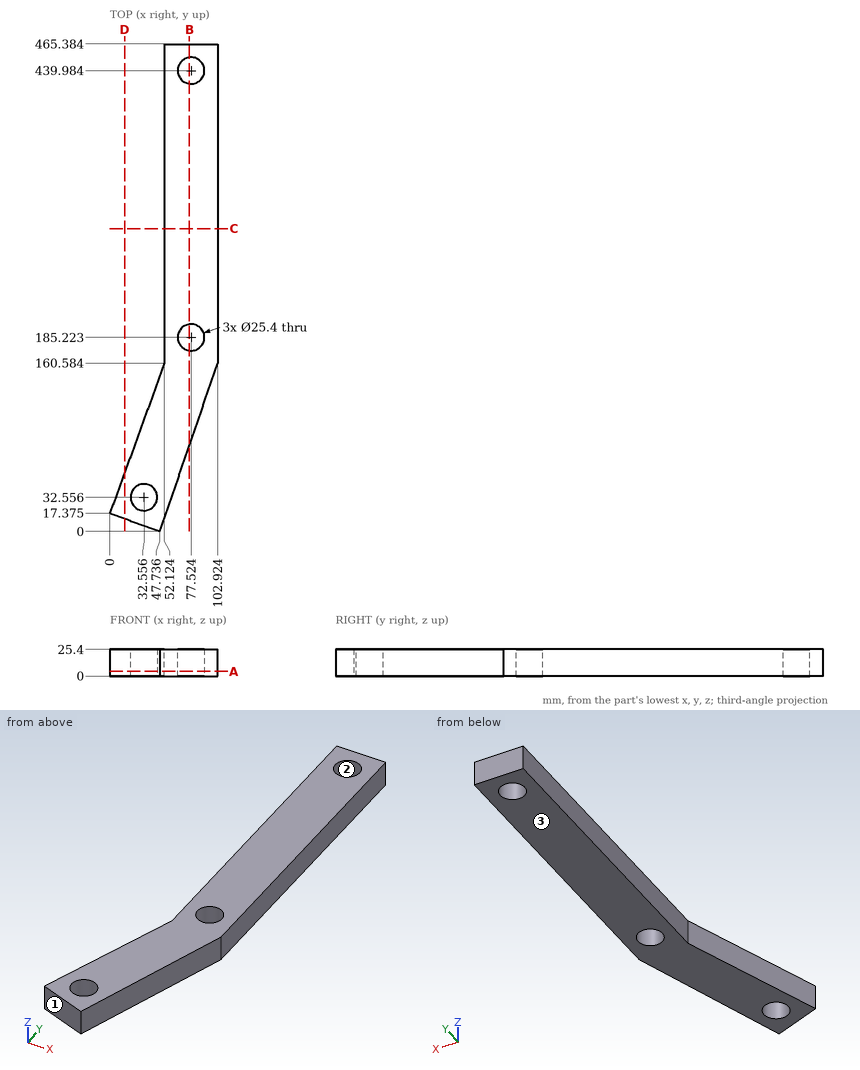
Drawing for the job (mm, zero at the part's lowest x, y, z). Coordinates: 2 decimals unless noted, no trailing zeros. Order: outer loops, then holes, each group sorted by start corner. A loop starts at its lowest first (then second) coordinate and runs counter-clockwise, first axis right, second up. Notation, with made-up numbers: (29.5, 13.5) -> (37.5, 13.5) arc R33 cw to (37.5, 47.5) -> close; hole circle Ø3 at (13.25, 72.5). An arc over 180 degrees is marked (long way). Return JSON: item names as keys, results as strings.
Item 1: Mould opens along X. For the marked faces 1, 2 and 3 say: pulls with the +X half, pulls with the -X half, needs draft (parallel to the pull), parting line crosses it, or undercut.
Model answer:
{"face 1": "pulls with the -X half", "face 2": "undercut", "face 3": "needs draft"}
Item 2: Slice it at D-D (x = 14). Write the cut outline in (y, z), then the cut area to 3 significant figures.
Model answer:
{"outline": "(12.28, 0) -> (55.84, 0) -> (55.84, 25.4) -> (12.28, 25.4) -> close", "area": "1,110 mm²"}
Item 3: Slice it at B-B (x = 76). Write the cut outline in (y, z) (1 decimal).
Model answer:
{"outline": "(82.2, 0) -> (172.6, 0) -> (172.6, 25.4) -> (82.2, 25.4) -> close; (197.8, 0) -> (427.4, 0) -> (427.4, 25.4) -> (197.8, 25.4) -> close; (452.6, 0) -> (465.4, 0) -> (465.4, 25.4) -> (452.6, 25.4) -> close"}
Item 4: Pin check, flat tips, straight feed: P1, Ø2, axis at y = 353.5, z = 15.5, coming from the -X side; P2, Ø3, axis at y = 141.5, z = 14, coming from the +X side. Stop position of each tip, or through.
Model answer:
{"P1": "stops at x = 52.12", "P2": "stops at x = 96.88"}
Item 5: Slice it at C-C (y = 289). Write the cut outline in (x, z).
Model answer:
{"outline": "(52.12, 0) -> (102.92, 0) -> (102.92, 25.4) -> (52.12, 25.4) -> close"}
Item 6: Wall check: line 1 along X through (y, z) = (325.5, 17.5); line 2 along X through (y, z) = (189.5, 23.75) (1 decimal); line 3 along X through (y, z) = (158.5, 7) (1 decimal). Give the ranges that are in metal, low to high. Write a range as from..to.
Model answer:
{"line 1": "x = 52.12..102.92", "line 2": "x = 52.1..65.6, 89.5..102.9", "line 3": "x = 51.4..102.2"}
Item 7: Slice it at A-A (z = 4.5). Write the cut outline in (x, y) (1 decimal).
Model answer:
{"outline": "(0, 17.4) -> (47.7, 0) -> (102.9, 160.6) -> (102.9, 465.4) -> (52.1, 465.4) -> (52.1, 160.6) -> close; hole circle Ø25.4 at (32.6, 32.6); hole circle Ø25.4 at (77.5, 185.2); hole circle Ø25.4 at (77.5, 440)"}
